Autodesk Inventor part; units mm, degrees
ref_plane "Work Plane2" through (-5.5, -7, 15) normal (0, 0, 1) x (1, 0, 0)
ref_plane "YZ Plane" through (0, 0, 0) normal (1, 0, 0) x (0, 1, 0)
ref_plane "XZ Plane" through (0, 0, 0) normal (0, 1, 0) x (-1, 0, 0)
sketch "Sketch1" plane through (0, 0, 0) normal (0, 0, 1) x (1, 0, 0)
  line L0 (-7.25, 10) -> (7.25, 10)
  line L1 (7.25, 10) -> (7.25, -10)
  line L2 (7.25, -10) -> (-7.25, -10)
  line L3 (-7.25, -10) -> (-7.25, 10)
  line L4 (0, 10) -> (0, -10) construction
  line L5 (-7.25, 0) -> (7.25, 0) construction
  line L6 (-1.75, 0) -> (1.75, 0) construction
  line L7 (-1.75, -2.75) -> (1.75, -2.75)
  line L8 (1.75, 2.75) -> (-1.75, 2.75)
  arc A0 (-1.75, 2.75) -> (-1.75, -2.75) centre (-1.75, 0) ccw
  arc A1 (1.75, -2.75) -> (1.75, 2.75) centre (1.75, 0) ccw
  point P0 (0, 0)
  point P1 (0, 0)
  dimension "d0" = 20
  dimension "d1" = 14.5
  dimension "d2" = 5.5
  dimension "d3" = 3.5
  dimension "d4" = 10
extrude "Extrusion1" add sketch "Sketch1" along normal blind 3
sketch "Sketch2" plane through (0, 0, 3) normal (0, 0, 1) x (1, 0, 0)
  line L0 (7.25, -10) -> (7.25, 10)
  line L1 (-7.25, -10) -> (7.25, -10)
  line L2 (7.25, -10) -> (7.25, -7)
  line L3 (7.25, -7) -> (-7.25, -7)
  line L4 (-7.25, -7) -> (-7.25, -10)
  point P0 (0, 0)
  dimension "d7" = 3
extrude "Extrusion2" add sketch "Sketch2" along normal blind 17
sketch "Sketch3" plane through (-7.25, -7, 3) normal (0, 1, 0) x (1, 0, 0)
  line L0 (0, 0) -> (0, -17)
  line L1 (14.5, -17) -> (0, -17)
  line L2 (14.5, 0) -> (14.5, -17)
  line L3 (0, -12) -> (14.5, -12) construction
  line L4 (4.5, -12) -> (10, -12) construction
  line L5 (4.5, -14.75) -> (10, -14.75)
  line L6 (10, -9.25) -> (4.5, -9.25)
  arc A0 (4.5, -9.25) -> (4.5, -14.75) centre (4.5, -12) ccw
  arc A1 (10, -14.75) -> (10, -9.25) centre (10, -12) ccw
  point P0 (7.25, 3)
  point P1 (7.25, -12)
  point P2 (7.25, -12)
  dimension "d10" = 5.5
  dimension "d11" = 5.5
  dimension "d12" = 5
extrude "Extrusion3" cut sketch "Sketch3" against normal up to surface (3 mm away)
ref_plane "Work Plane2" through (-5.5, -7, 15) normal (0, 0, 1) x (1, 0, 0)
ref_plane "Work Plane3" through (0, -10, 0) normal (1, 0, 0) x (0, 0, -1)
properties part number "L bracket single"
Source: CAD feature listing. Evaluate the final solid. Frame: model axes, mm. A direction names the side the tool comes from. Round coordinates to 2 decimals unless told otherwise and drop trailing zeros. Loops run counter-clockwise (first coordinate to the right, second up) from the corner with the lowest first, then second, coordinate; pieces in that order, holes last.
1. Contact query for flat-ended pins moving along their axis: pin 1 (8 mm diameter, centred on x = 4, z = 12, fed in from +Y); pin 2 (6 mm diameter, centred on x = -3.5, y = 3, fed in from +Z); pin 3 (1 mm diameter, centred on x = 1, z = 13, fed in from +Y). Output: stop coordinate, or through.
2. Ray query, L1, parallel to Z at x = -2.75, y = -7.5; L2, parallel to Y at x = -3.5, z = 10.75; L3, parallel to Z at x = 3, y = -7.25. Return the intervals inside material, ascending.
3. Section query B-B on x = -1. Output: boundary loops of the cut face in (y, z), and give its area (3 significant figures).
4. Access query for faces 1 (the flat face through (7.25, -4.4, 2.5)), 2 (the cylindrical face through (5.5, -8.5, 15.1)), 3 (the flat face through (0, 4, 3)), 4 (the flat face through (0, 2.75, 1)). Directions: +Z, -Z, +X, -X, +Y, -Y. A direction counts if a zero-diameter tool reaches every point of the face in a straight line with its end or side. Return the directions, or none.
5. Section query D-D on z = 6. Output: boundary loops of the cut face in (x, y), and give its area (3 significant figures).
6. Section query C-C on y = -1.25. Output: boundary loops of the cut face in (x, z), and give its area (3 significant figures).
7. Section query A-A on z = 15. Output: boundary loops of the cut face in (x, y).
8. Mould query, pull axis X, two halves, no side actions, for faces 5 (the flat face through (0, -7, 9)), 6 (the flat face through (0, -2.75, 1)), 7 (the flat face through (0, -8, 17.75)), 8 (the flat face through (-7.25, -4.5, 2.5)). Classes: released by +X, released by -X, zero draft, split by the parting line, or undercut.
Answers below:
1. pin 1: stops at y = -7
1. pin 2: stops at z = 3
1. pin 3: passes through
2. L1: z = 0 to 12.25, 17.75 to 20
2. L2: y = -10 to -7
2. L3: z = 0 to 12.26, 17.74 to 20
3. outline: (-10, 0) - (-2.75, 0) - (-2.75, 3) - (-7, 3) - (-7, 12.25) - (-10, 12.25) - close; (-10, 17.75) - (-7, 17.75) - (-7, 20) - (-10, 20) - close; (2.75, 0) - (10, 0) - (10, 3) - (2.75, 3) - close
3. area: 78.0 mm2
4. face 1: +Z, -Z, +X, +Y, -Y
4. face 2: +Y, -Y
4. face 3: +Z, +X, -X, +Y
4. face 4: +Z, -Z
5. outline: (-7.25, -10) - (7.25, -10) - (7.25, -7) - (-7.25, -7) - close
5. area: 43.5 mm2
6. outline: (-7.25, 0) - (-4.2, 0) - (-4.2, 3) - (-7.25, 3) - close; (4.2, 0) - (7.25, 0) - (7.25, 3) - (4.2, 3) - close
6. area: 18.3 mm2
7. outline: (-7.25, -10) - (-5.5, -10) - (-5.5, -7) - (-7.25, -7) - close; (5.5, -10) - (7.25, -10) - (7.25, -7) - (5.5, -7) - close
8. face 5: zero draft
8. face 6: undercut
8. face 7: undercut
8. face 8: released by -X
